from build123d import *

# Parameters (mm, degrees)
EXTRUDE_1_DEPTH        = 1.6
SKETCH_2_W             = 23.2
SKETCH_2_H             = 6
EXTRUDE_719_DEPTH      = 1.6
CUT_EXTRUDE_1150_REACH = 43.724
SKETCH_5_R             = 2.6
CUT_EXTRUDE_1612_DEPTH = 1
CUT_EXTRUDE_1748_REACH = 43.864
SKETCH_7_R             = 1.25
SKETCH_9_W             = 36
SKETCH_9_H             = 22
CUT_EXTRUDE_2286_DEPTH = 0.6
FILLET_2_R             = 1


with BuildPart() as part:
    # 草图1 → 凸台-拉伸1 (new body)
    with BuildSketch(Plane(origin=(0, 0, 0), x_dir=(1, 0, 0), z_dir=(0, 1, 0))):
        with BuildLine():
            Line((-33.1, -22), (33.1, -22))
            Line((33.1, -22), (33.1, 19))
            ThreePointArc((33.1, 19), (32.221320344, 21.121320344), (30.1, 22))
            Line((30.1, 22), (-30.1, 22))
            ThreePointArc((-30.1, 22), (-32.221320344, 21.121320344), (-33.1, 19))
            Line((-33.1, 19), (-33.1, -22))
        make_face()
    extrude(amount=EXTRUDE_1_DEPTH)

    # 草图2 → Extrude 719 (add)
    with BuildSketch(Plane.XY.offset(22)):
        with BuildLine():
            Line((-33.1, 0), (33.1, 0))
            Line((33.1, 0), (33.1, 10))
            ThreePointArc((33.1, 10), (32.807106781, 10.707106781), (32.1, 11))
            Line((32.1, 11), (17.1, 11))
            Line((17.1, 11), (-9.1, 11))
            Line((-9.1, 11), (-32.1, 11))
            ThreePointArc((-32.1, 11), (-32.807106781, 10.707106781), (-33.1, 10))
            Line((-33.1, 10), (-33.1, 0))
        make_face()
        with Locations((3.5, 7)):
            Rectangle(SKETCH_2_W, SKETCH_2_H, mode=Mode.SUBTRACT)
    extrude(amount=EXTRUDE_719_DEPTH)

    # 草图3 → Cut-Extrude 1150 (cut, up to next)
    with BuildSketch(Plane(origin=(0, 1.6, 0), x_dir=(1, 0, 0), z_dir=(0, 1, 0)), mode=Mode.PRIVATE) as cut_extrude_1150_sk1:
        with BuildLine():
            Line((-8.5, -7), (11.5, -7))
            ThreePointArc((11.5, -7), (12.914213562, -6.414213562), (13.5, -5))
            Line((13.5, -5), (13.5, 5))
            ThreePointArc((13.5, 5), (12.914213562, 6.414213562), (11.5, 7))
            Line((11.5, 7), (-8.5, 7))
            ThreePointArc((-8.5, 7), (-9.914213562, 6.414213562), (-10.5, 5))
            Line((-10.5, 5), (-10.5, -5))
            ThreePointArc((-10.5, -5), (-9.914213562, -6.414213562), (-8.5, -7))
        make_face()
    cut_extrude_1150_tool1 = extrude(cut_extrude_1150_sk1.sketch, amount=-CUT_EXTRUDE_1150_REACH, mode=Mode.PRIVATE) & part.part
    add(cut_extrude_1150_tool1.solids().sort_by_distance((1.5, 1.6, 0))[0], mode=Mode.SUBTRACT)

    # 草图5 → Cut-Extrude 1612 (cut)
    with BuildSketch(Plane.XZ):
        with Locations(Location((-28, -16.9, 0), (0, 0, 270))):
            Circle(SKETCH_5_R)
        with Locations(Location((28, -16.9, 0), (0, 0, 270))):
            Circle(SKETCH_5_R)
        with Locations(Location((28, 18.1, 0), (0, 0, 270))):
            Circle(SKETCH_5_R)
        with Locations(Location((-28, 18.1, 0), (0, 0, 270))):
            Circle(SKETCH_5_R)
    extrude(amount=-CUT_EXTRUDE_1612_DEPTH, mode=Mode.SUBTRACT)

    # 草图7 → Cut-Extrude 1748 (cut, up to next)
    with BuildSketch(Plane.XZ.offset(-1), mode=Mode.PRIVATE) as cut_extrude_1748_sk1:
        with Locations(Location((-28, -16.9, 0), (0, 0, 270))):
            Circle(SKETCH_7_R)
    cut_extrude_1748_tool1 = extrude(cut_extrude_1748_sk1.sketch, amount=-CUT_EXTRUDE_1748_REACH, mode=Mode.PRIVATE) & part.part
    # 草图7 → Cut-Extrude 1748 (cut, up to next)
    with BuildSketch(Plane.XZ.offset(-1), mode=Mode.PRIVATE) as cut_extrude_1748_sk2:
        with Locations(Location((28, -16.9, 0), (0, 0, 270))):
            Circle(SKETCH_7_R)
    cut_extrude_1748_tool2 = extrude(cut_extrude_1748_sk2.sketch, amount=-CUT_EXTRUDE_1748_REACH, mode=Mode.PRIVATE) & part.part
    # 草图7 → Cut-Extrude 1748 (cut, up to next)
    with BuildSketch(Plane.XZ.offset(-1), mode=Mode.PRIVATE) as cut_extrude_1748_sk3:
        with Locations(Location((28, 18.1, 0), (0, 0, 270))):
            Circle(SKETCH_7_R)
    cut_extrude_1748_tool3 = extrude(cut_extrude_1748_sk3.sketch, amount=-CUT_EXTRUDE_1748_REACH, mode=Mode.PRIVATE) & part.part
    # 草图7 → Cut-Extrude 1748 (cut, up to next)
    with BuildSketch(Plane.XZ.offset(-1), mode=Mode.PRIVATE) as cut_extrude_1748_sk4:
        with Locations(Location((-28, 18.1, 0), (0, 0, 270))):
            Circle(SKETCH_7_R)
    cut_extrude_1748_tool4 = extrude(cut_extrude_1748_sk4.sketch, amount=-CUT_EXTRUDE_1748_REACH, mode=Mode.PRIVATE) & part.part
    add(cut_extrude_1748_tool1.solids().sort_by_distance((-28, 1, -16.9))[0], mode=Mode.SUBTRACT)
    add(cut_extrude_1748_tool2.solids().sort_by_distance((28, 1, -16.9))[0], mode=Mode.SUBTRACT)
    add(cut_extrude_1748_tool3.solids().sort_by_distance((28, 1, 18.1))[0], mode=Mode.SUBTRACT)
    add(cut_extrude_1748_tool4.solids().sort_by_distance((-28, 1, 18.1))[0], mode=Mode.SUBTRACT)

    # 草图9 → Cut-Extrude 2286 (cut)
    with BuildSketch(Plane(origin=(0, 1.6, 0), x_dir=(1, 0, 0), z_dir=(0, 1, 0))):
        with Locations((1.500900608, 0.362797629)):
            Rectangle(SKETCH_9_W, SKETCH_9_H)
    extrude(amount=-CUT_EXTRUDE_2286_DEPTH, mode=Mode.SUBTRACT)

    # 圆角2
    fillet_2_edges = [part.edges().sort_by_distance(p)[0] for p in [
        (32.807106781, 10.707106781, 23.6),
        (0, 11, 23.6),
        (-32.807106781, 10.707106781, 23.6),
        (-33.1, 5, 23.6),
        (33.1, 5, 23.6),
    ]]
    fillet(fillet_2_edges, radius=FILLET_2_R - 0.0001)  # a hair under: the kernel refuses the full size


solid = part.part
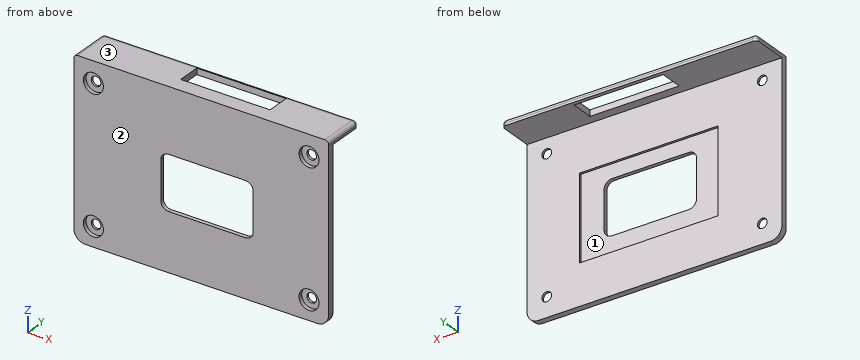
Model file for the job. Use its own axes, mm. Face numbers are marked on the shaded views. Coordinates: 2 decimals unless noted, no trailing zeros. Order: outer loops, then holes, each group sorted by start corner. A loop starts at its lowest first (then second) coordinate and runs counter-clockwise, first axis right, second up. Notation, with made-up numbers: M 88,-28.5 L 111,-28.5 A20 cw 111,8.5 Z; hole C 40,-34.5 d7. An arc over 180 degrees is marked long. Return JSON: item names as keys, results as strings.
1. Saw through at A-A (x = 10.5). Give the number of separate pieces and of enclosed holes in the cut face, and give its area (3 significant figures).
Ans:
{"separate pieces": "3", "enclosed holes": "0", "area": "51.0 mm^2"}
2. Pull direction Z, two halves, no side cores. Call the marked faces 1, 2 and 3: +Z half, -Z half, draft (parallel to the pull), parting line (faces both ways), or undercut.
Ans:
{"face 1": "undercut", "face 2": "draft", "face 3": "+Z half"}
3. Drill centre lines: probe 1 along X at (y, z) = (1.55, 18.1); probe 2 along Z at (x, y) = (22, 4.25); probe 3 along Y at (x, z) = (11.5, 9.5). Where is each one in solid material? Low to high.
Ans:
{"probe 1": "-33.1 to -29.25, -26.75 to 26.75, 29.25 to 33.1", "probe 2": "22 to 23.6", "probe 3": "0 to 1"}
4. Flat gauge pins, fed straight in: pin 1 (1.6 mm diameter, centred on x = -27, z = 19, fed in from -Y); pin 2 (10 mm diameter, centred on x = -3, z = -3.5, fed in from +Y); pin 3 (2 mm diameter, centred on x = 7, z = -17, fed in from +Y). Where does each tip first touch, or does it go through?
Ans:
{"pin 1": "y = 1", "pin 2": "y = 1", "pin 3": "y = 1.6"}
5. Saw through at B-B (z = -16.9). Give the cut face in (x, y).
Ans:
{"outline": "M -33.1,0 L -30.6,0 L -30.6,1 L -29.25,1 L -29.25,1.6 L -33.1,1.6 Z; M -26.75,1 L -25.4,1 L -25.4,0 L 25.4,0 L 25.4,1 L 26.75,1 L 26.75,1.6 L -26.75,1.6 Z; M 29.25,1 L 30.6,1 L 30.6,0 L 33.1,0 L 33.1,1.6 L 29.25,1.6 Z"}
6. Saw through at C-C (y = 5.25). Give the cut face in (x, z).
Ans:
{"outline": "M -33.1,22 L -8.1,22 L -8.1,23.6 L -32.1,23.6 A1 ccw -33.1,22.6 Z; M 15.1,22 L 33.1,22 L 33.1,22.6 A1 ccw 32.1,23.6 L 15.1,23.6 Z"}
7. Saw through at D-D (z = 1.5). Give the cut face in (x, y), and give its area (3 significant figures).
Ans:
{"outline": "M -33.1,0 L -10.5,0 L -10.5,1 L -16.5,1 L -16.5,1.6 L -33.1,1.6 Z; M 13.5,0 L 33.1,0 L 33.1,1.6 L 19.5,1.6 L 19.5,1 L 13.5,1 Z", "area": "60.3 mm^2"}
